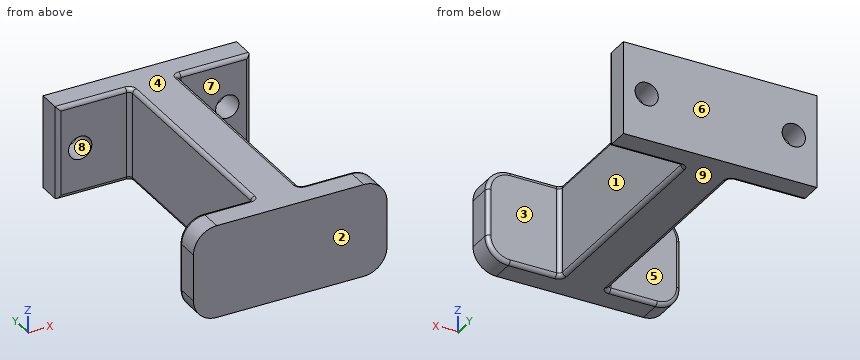
```python
from build123d import *

# Parameters (mm, degrees)
BOSS_EXTRUDE1_DEPTH = 6
FILLET1_R           = 3
CUT_EXTRUDE1_REACH  = 39.646
SKETCH2_R           = 1.5
FILLET2_R           = 0.5


with BuildPart() as part:
    # Sketch1 → Boss-Extrude1 (new, symmetric)
    with BuildSketch(Plane.XY):
        Polygon((0, 0), (-12.5, 0), (-12.5, 3.25), (-3, 3.25), (-3, 31.75), (-12.5, 31.75), (-12.5, 35), (12.5, 35), (12.5, 31.75), (3, 31.75), (3, 3.25), (12.5, 3.25), (12.5, 0), align=None)
    extrude(amount=BOSS_EXTRUDE1_DEPTH, both=True)

    # Fillet1
    fillet1_edges = [part.edges().sort_by_distance(p)[0] for p in [
        (-12.5, 1.625, -6),
        (12.5, 1.625, -6),
        (-12.5, 1.625, 6),
        (12.5, 1.625, 6),
    ]]
    fillet(fillet1_edges, radius=FILLET1_R)

    # Sketch2 → Cut-Extrude1 (cut, up to next)
    with BuildSketch(Plane(origin=(0, 35, 0), x_dir=(1, 0, 0), z_dir=(0, 1, 0)), mode=Mode.PRIVATE) as cut_extrude1_sk1:
        with Locations(Location((-9.5, 0, 0), (0, 0, 270))):
            Circle(SKETCH2_R)
    cut_extrude1_tool1 = extrude(cut_extrude1_sk1.sketch, amount=-CUT_EXTRUDE1_REACH, mode=Mode.PRIVATE) & part.part
    # Sketch2 → Cut-Extrude1 (cut, up to next)
    with BuildSketch(Plane(origin=(0, 35, 0), x_dir=(1, 0, 0), z_dir=(0, 1, 0)), mode=Mode.PRIVATE) as cut_extrude1_sk2:
        with Locations(Location((9.5, 0, 0), (0, 0, 270))):
            Circle(SKETCH2_R)
    cut_extrude1_tool2 = extrude(cut_extrude1_sk2.sketch, amount=-CUT_EXTRUDE1_REACH, mode=Mode.PRIVATE) & part.part
    add(cut_extrude1_tool1.solids().sort_by_distance((-9.5, 35, 0))[0], mode=Mode.SUBTRACT)
    add(cut_extrude1_tool2.solids().sort_by_distance((9.5, 35, 0))[0], mode=Mode.SUBTRACT)

    # Fillet2
    fillet2_edges = [part.edges().sort_by_distance(p)[0] for p in [
        (-6.25, 3.25, -6),
        (-3, 17.5, -6),
        (-7.75, 31.75, -6),
        (7.75, 31.75, -6),
        (3, 17.5, -6),
        (3, 17.5, 6),
        (7.75, 31.75, 6),
        (-3, 3.25, 0),
        (-3, 31.75, 0),
        (-12.5, 31.75, 0),
        (12.5, 31.75, 0),
        (3, 31.75, 0),
        (3, 3.25, 0),
        (-7.75, 31.75, 6),
        (-12.5, 3.25, 0),
        (-3, 17.5, 6),
        (-6.25, 3.25, 6),
        (6.25, 3.25, -6),
        (-11.621320344, 3.25, 5.121320344),
        (-11.621320344, 3.25, -5.121320344),
        (12.5, 3.25, 0),
        (6.25, 3.25, 6),
        (11.621320344, 3.25, 5.121320344),
        (11.621320344, 3.25, -5.121320344),
    ]]
    fillet(fillet2_edges, radius=FILLET2_R)


solid = part.part
```
Verification items for the finished model (mm, model axes). Face numbers are marked on the shaded views. A direction names the side the tool comes from. Coordinates: 2 decimals unless noted, no trailing zeros. Write each loop counter-clockwise with the first axis right and the second up, starting at its lowest first coordinate (ties: lowest second). Pieces come first, ordered by that corner, then holes. Notation, with made-up numbers: M -3,-3 L 23,-3 A13 ccw 23,9 Z; hole C 68,59.5 d3. An arc over 180 degrees is marked long. One line per item, written item: value.
Item 1: Gauge pin test, flat ends, axial feed: pin 1 Ø1 at (y, z) = (11, -3) entering from +X; pin 2 Ø2.5 at (x, z) = (-9.5, 0) entering from +Y. Record the tip position at first contact, or that the pin passes through.
Check sheet entries:
pin 1: stops at x = 3
pin 2: stops at y = 3.25
Item 2: Section check B-B, the plane z = 0. Record the boundary of the cut face in (x, y).
Check sheet entries:
outline: M -12.5,0 L 12.5,0 L 12.5,2.75 A0.5 ccw 12,3.25 L 3.5,3.25 A0.5 cw 3,3.75 L 3,31.25 A0.5 cw 3.5,31.75 L 8,31.75 L 8,35 L -8,35 L -8,31.75 L -3.5,31.75 A0.5 cw -3,31.25 L -3,3.75 A0.5 cw -3.5,3.25 L -12,3.25 A0.5 ccw -12.5,2.75 Z; M -12.5,32.25 A0.5 ccw -12,31.75 L -11,31.75 L -11,35 L -12.5,35 Z; M 11,31.75 L 12,31.75 A0.5 ccw 12.5,32.25 L 12.5,35 L 11,35 Z
Item 3: Mould release check, pull along Y, two halves, no side actions. Record for the marked faces 1, 2, 3 and 4: pulls with the +Y half, pulls with the -Y half, needs draft (parallel to the pull), parting line crosses it, or undercut.
Check sheet entries:
face 1: undercut
face 2: pulls with the -Y half
face 3: undercut
face 4: needs draft
Item 4: Access from +Z, -Z, +X, -X, +Y, -Y to the whole of each face (thin tool, end or side, straight path). Record for the marked faces 5, 6, 7, 8 and 9.
Check sheet entries:
face 5: +Z, -Z, -X
face 6: +Z, -Z, +X, -X, +Y
face 7: +Z, -Z, +X
face 8: +Y
face 9: -Z, +X, -X, +Y, -Y
Item 5: Section check A-A, the plane x = -7.5. Record the boundary of the cut face in (y, z), plus the area to 3 significant figures.
Check sheet entries:
outline: M 0,-6 L 2.75,-6 A0.5 ccw 3.25,-5.5 L 3.25,5.5 A0.5 ccw 2.75,6 L 0,6 Z; M 31.75,-5.5 A0.5 ccw 32.25,-6 L 35,-6 L 35,6 L 32.25,6 A0.5 ccw 31.75,5.5 Z
area: 77.8 mm^2
Item 6: Section check C-C, the plane y = 20.5. Record the boundary of the cut face in (x, z), plus the area to 3 significant figures.
Check sheet entries:
outline: M -3,-5.5 A0.5 ccw -2.5,-6 L 2.5,-6 A0.5 ccw 3,-5.5 L 3,5.5 A0.5 ccw 2.5,6 L -2.5,6 A0.5 ccw -3,5.5 Z
area: 71.8 mm^2
Item 7: Scan lines: line 1 along X through (y, z) = (32.95, 0); line 2 along Y through (x, z) = (-5.5, 2); line 3 along X through (y, z) = (26.5, 2.5). Record each from-to range of solid material in increasing order.
Check sheet entries:
line 1: x = -12.5 to -11, -8 to 8, 11 to 12.5
line 2: y = 0 to 3.25, 31.75 to 35
line 3: x = -3 to 3
Item 8: Section check D-D, the plane y = 33. Record the boundary of the cut face in (x, z).
Check sheet entries:
outline: M -12.5,-6 L 12.5,-6 L 12.5,6 L -12.5,6 Z; hole C -9.5,0 d3; hole C 9.5,0 d3
